from build123d import *

# Parameters (mm, degrees)
F1_ANGLE_BACK = 90
F1_ANGLE      = 180
F2_R          = 2.5
F3_DEPTH      = 28.501
F3_DEPTH_BACK = 28.501
F4_R          = 1.905
F5_W          = 6
F5_H          = 2.5
F5_W_2        = 45
F5_H_2        = 6
F5_H_3        = 1.5
F6_DEPTH      = 6


with BuildPart() as f1:
    # F0 (on Front) → F1 (revolve)
    with BuildSketch(Plane.XZ, mode=Mode.PRIVATE) as f1_sk:
        Polygon((-18.5, 0), (0, 0), (0, 10), (-18.5, 10), (-18.5, 50), (-10, 50), (-10, 60), (-18.5, 60), (-28.5, 60), (-28.5, 0), align=None)
    revolve(f1_sk.sketch.rotate(Axis((0, 0, 5), (0, 0, 1)), -F1_ANGLE_BACK), axis=Axis((0, 0, 5), (0, 0, 1)), revolution_arc=F1_ANGLE)

    # F2 (on Front) → F3 (cut, two sides)
    with BuildSketch(Plane.XZ) as f3_sk:
        with Locations((0, 60)):
            Circle(F2_R)
    extrude(amount=-F3_DEPTH, mode=Mode.SUBTRACT)
    extrude(f3_sk.sketch, amount=F3_DEPTH_BACK, mode=Mode.SUBTRACT)

    # F4
    f4_edges = [f1.edges().sort_by_distance(p)[0] for p in [
        (-18.5, 0, 10),
    ]]
    fillet(f4_edges, radius=F4_R)

    # F5 (on face) → F6 (cut)
    with BuildSketch(Plane.YZ):
        with Locations((-25.5, 58.75)):
            Rectangle(F5_W, F5_H)
        Polygon((-22.5, 6), (-22.5, 56), (-28.5, 56), (-28.5, 0), (-22.5, 0), align=None)
        with Locations((25.5, 58.75)):
            Rectangle(F5_W, F5_H)
        Polygon((22.5, 56), (22.5, 6), (22.5, 0), (28.5, 0), (28.5, 56), align=None)
        with Locations((0, 3)):
            Rectangle(F5_W_2, F5_H_2)
        with Locations((25.5, 56.75)):
            Rectangle(F5_W, F5_H_3)
        with Locations((-25.5, 56.75)):
            Rectangle(F5_W, F5_H_3)
    extrude(amount=-F6_DEPTH, mode=Mode.SUBTRACT)


solid = f1.part
Read the model definition and answer for the solid it produces. Units are mm, in the model's axes. A direction names the side the tool comes from. Round coordinates to 2 decimals unless told otherwise and drop trailing zeros. Loops run counter-clockwise (first coordinate to the right, second up) from the corner with the lowest first, then second, coordinate; pieces in that order, holes last. Notation, with made-up numbers: (86.5, 60.5) - (99.5, 60.5) arc R33 cw to (99.5, 88.5) - close; hole circle Ø9 at (70.25, -22.5). An arc over 180 degrees is marked (long way). One line per question, with ' | ' between items. Start each with the question number.
Q1. Section C-C on z = 30.5 is taken. Give the vertices of the cut face in (x, y), plus the area to 3 significant figures.
Q2. Flat-ended cylindrical pins translate along their axes: pin 1 (5 mm diameter, centred on x = -3, y = -2.5, fed in from -Z); pin 2 (1.5 mm diameter, centred on x = -21, z = 49, fed in from -Y); pin 3 (1.5 mm diameter, centred on x = -25, z = 51.5, fed in from +Y). Find the tip coordinate at first contact, or state that the pin passes through.
Q3. Section B-B on y = 0 is taken. Give the vertices of the cut face in (x, z) (3 decimals).
Q4. Section A-A on z = 55.5 is taken. Give the vertices of the cut face in (x, y), plus the area to 3 significant figures.
Q5. Section D-D on x = -21.5 is taken. Give the vertices of the cut face in (y, z), plus the area to 4 significant figures.
Q6. For a pull along Y with two mould halves and no side action, classify faces 1 (the flat face through (-3, 22.5, 33)), 2 (the cylindrical face through (-18.496, 0.407, 31.219)), 3 (the flat face through (-3, -22.5, 33)), 4 (the flat face through (-3, 0, 6)) as +Y half, -Y half, draft (parallel to the pull), parting line (faces both ways), or undercut.
Q7. For faces 5 (the flat face through (-7, 0, 10)), 6 (the cylindrical face through (-10, 0, 55)), 7 (the cylindrical face through (-1.787, 16.002, 58.252)), determine the directions among +Z, -Z, +X, -X, +Y, -Y from which every point of the face is accessible in a straight line to the end or side of a thin tool.
Q8. Find the intervals of material crossed by L1, parallel to Z at x = -4, y = -10.5; L2, parallel to Z at x = -7.5, y = 12.5; L3, parallel to Y at x = -1.25, z = 54, in increasing order.
Established:
1) outline: (-6, -27.86) - (-6, -22.5) - (0, -22.5) - (0, -18.5) arc R18.5 cw to (0, 18.5) - (0, 22.5) - (-6, 22.5) - (-6, 27.86) arc R28.5 ccw to start | area: 669 mm²
2) pin 1: z = 6 | pin 2: y = -20.05 | pin 3: y = 14.97
3) outline: (-28.5, 0) - (-6, 0) - (-6, 6) - (0, 6) - (0, 10) - (-16.595, 10) arc R1.905 cw to (-18.5, 11.905) - (-18.5, 50) - (-10, 50) - (-10, 60) - (-28.5, 60) - close
4) outline: (-6, -27.86) - (-6, -22.5) - (0, -22.5) - (0, -10) arc R10 cw to (0, 10) - (0, 22.5) - (-6, 22.5) - (-6, 27.86) arc R28.5 ccw to start | area: 1,050 mm²
5) outline: (-18.71, 0) - (18.71, 0) - (18.71, 60) - (-18.71, 60) - close | area: 2,245 mm²
6) face 1: +Y half | face 2: undercut | face 3: -Y half | face 4: draft
7) face 5: +X | face 6: +Z, +X | face 7: +Z, +X, +Y, -Y
8) L1: 6 to 10, 50 to 60 | L2: 0 to 10, 50 to 60 | L3: -22.5 to -9.92, 9.92 to 22.5
